Autodesk Inventor part; units mm, degrees
ref_plane "YZ Plane" through (0, 0, 0) normal (1, 0, 0) x (0, 1, 0)
ref_plane "XZ Plane" through (0, 0, 0) normal (0, 1, 0) x (-1, 0, 0)
ref_plane "XY Plane" through (0, 0, 0) normal (0, 0, 1) x (1, 0, 0)
sketch "Sketch1" plane through (0, 0, 0) normal (0, 0, 1) x (1, 0, 0)
  line L0 (0, 0) -> (25.4, 0)
  line L1 (25.4, 0) -> (25.4, 25.4)
  line L2 (25.4, 25.4) -> (0, 25.4)
  line L3 (0, 25.4) -> (0, 0)
  circle A0 centre (12.7, 12.7) radius 3.175
  dimension "d0" = 25.4
  dimension "d1" = 25.4
  dimension "d2" = 6.35
  dimension "d7" = 12.7
  dimension "d8" = 12.7
extrude "Extrusion1" add sketch "Sketch1" along normal blind 609.6
sketch "Sketch2" plane through (0, 0, 609.6) normal (0, 0, 1) x (1, 0, 0)
  line L0 (25.4, 25.4) -> (0, 25.4)
  line L1 (0, 25.4) -> (0, 0)
  circle A0 centre (12.7, 12.7) radius 3.175
  line L2 (0, 0) -> (25.4, 0)
  line L3 (25.4, 0) -> (25.4, 25.4)
  line L4 (25.4, 25.4) -> (0, 25.4)
  line L5 (0, 25.4) -> (0, 0)
  line L6 (12.7, 19.05) -> (9.525, 19.05)
  line L7 (9.525, 19.05) -> (15.875, 19.05)
  line L8 (15.875, 19.05) -> (19.05, 25.4)
  line L9 (9.525, 19.05) -> (6.35, 25.4)
  dimension "d13" = 6.35
  dimension "d14" = 6.35
  dimension "d15" = 3.175
  dimension "d16" = 6.35
fillet "Fillet1" radius 1.5875 4 edges at (25.4, 25.4, 304.8) (0, 25.4, 304.8) (25.4, 0, 304.8) (0, 0, 304.8)
extrude "Extrusion2" cut sketch "Sketch2" against normal blind 609.6 contours L8 L7 L6 L9 L0
pattern_circular "Circular Pattern1" count 4 over 360 about axis through (12.7, 12.7, 0) along (0, 0, 1) of "Extrusion2"
sketch "Sketch3" plane through (0, 0, 609.6) normal (0, 0, 1) x (1, 0, 0)
  line L0 (19.05, 15.875) -> (25.4, 19.05)
  line L1 (25.4, 19.05) -> (25.4, 23.8125)
  arc A0 (25.4, 23.8125) -> (23.8125, 25.4) centre (23.8125, 23.8125) ccw
  line L2 (23.8125, 25.4) -> (19.05, 25.4)
  line L3 (19.05, 25.4) -> (15.875, 19.05)
  line L4 (15.875, 19.05) -> (9.525, 19.05)
  line L5 (9.525, 19.05) -> (6.35, 25.4)
  line L6 (6.35, 25.4) -> (1.5875, 25.4)
  arc A1 (1.5875, 25.4) -> (0, 23.8125) centre (1.5875, 23.8125) ccw
  line L7 (0, 23.8125) -> (0, 19.05)
  line L8 (0, 19.05) -> (6.35, 15.875)
  line L9 (6.35, 15.875) -> (6.35, 9.525)
  line L10 (6.35, 9.525) -> (0, 6.35)
  line L11 (0, 6.35) -> (0, 1.5875)
  arc A2 (0, 1.5875) -> (1.5875, 0) centre (1.5875, 1.5875) ccw
  line L12 (1.5875, 0) -> (6.35, 0)
  line L13 (6.35, 0) -> (9.525, 6.35)
  line L14 (9.525, 6.35) -> (15.875, 6.35)
  line L15 (15.875, 6.35) -> (19.05, 0)
  line L16 (19.05, 0) -> (23.8125, 0)
  arc A3 (23.8125, 0) -> (25.4, 1.5875) centre (23.8125, 1.5875) ccw
  line L17 (25.4, 1.5875) -> (25.4, 6.35)
  line L18 (25.4, 6.35) -> (19.05, 9.525)
  line L19 (19.05, 9.525) -> (19.05, 15.875)
  circle A4 centre (12.7, 12.7) radius 3.175
  point P0 (0, 0)
extrude "Extrusion3" cut sketch "Sketch3" against normal blind 517.525
properties part number "Mock 8020 3.625in"
Design review of the part built by this model. Coordinates are the model's own, in mm. A direction names the side the tool comes from. Round coordinates to 2 decimals unless told otherwise and drop trailing zeros. Loops run counter-clockwise (first coordinate to the right, second up) from the corner with the lowest first, then second, coordinate; pieces in that order, holes last. Notation, with made-up numbers: (-35, -5.5) - (-16, -5.5) arc R18 cw to (-16, 9.5) - close; hole circle Ø4 at (47, -10.5). An arc over 180 degrees is marked (long way). One line per item, written item: value. Start each with the question number.
1) Insertion check: pin 1 Ø5 at (x, z) = (14, 30.5) entering from -Y; pin 2 Ø1.9 at (y, z) = (11.5, 53.5) entering from +X; pin 3 Ø1 at (x, z) = (7, 21.5) entering from -Y; pin 4 Ø3 at (x, z) = (3.5, 51.5) entering from -Y. Each pin has a flat end and moves straight along its axis. Give the tip position at first contact, or say it passes through.
2) Consider section A-A on y = 21. Give the boundary of the cut face in (x, z) (3 decimals), then the cut area to 3 significant figures.
3) To check wall thickness, follow L1, parallel to Y at x = 12.7, z = 58.5 (3 decimals); L2, parallel to X at y = 6, z = 86.5; L3, parallel to Y at x = 15.5, z = 41.5. State the ranges of each line that lie inside material, in increasing order. Write a range as from..to.
4) Consider section C-C on x = 12.7. Give the boundary of the cut face in (y, z) (3 decimals).
5) For faces 1 (the flat face through (3.22, 17.44, 46.68)), 2 (the flat face through (0, 4, 45)), 3 (the flat face through (7.96, 22.18, 46.68)), 4 (the flat face through (19.05, 13, 47)), list the 3-axis set-ups (+Z, -Z, +X, -X, +Y, -Y) from which the entire face can be reached by the end or side of a thin tool; tool diameter is ignored.
6) Consider section D-D on y = 7.5. Give the boundary of the cut face in (x, z) (3 decimals), then the cut area to 3 significant figures.
7) Draft analysis for pull direction X (two halves, no side actions). For faces 5 (the flat face through (0, 21, 45)), 6 (the flat face through (4, 25.4, 45)), 7 (the flat face through (17.44, 3.22, 46.68)), state which applies: +X half, -X half, draft (parallel to the pull), parting line (faces both ways), or undercut.
Reported:
1. pin 1: stops at y = 5.1
1. pin 2: stops at x = 19.05
1. pin 3: stops at y = 0.3
1. pin 4: stops at y = 0
2. outline: (0, 0) - (8.55, 0) - (8.55, 92.075) - (0, 92.075) - close; (16.85, 0) - (25.4, 0) - (25.4, 92.075) - (16.85, 92.075) - close
2. area: 1,570 mm^2
3. L1: y = 6.35..9.525, 15.875..19.05
3. L2: x = 0..9.35, 16.05..25.4
3. L3: y = 6.35..11.2, 14.2..19.05
4. outline: (6.35, 0) - (9.525, 0) - (9.525, 92.075) - (6.35, 92.075) - close; (15.875, 0) - (19.05, 0) - (19.05, 92.075) - (15.875, 92.075) - close
5. face 1: +Z, -Z, -X
5. face 2: +Z, -Z, -X, +Y, -Y
5. face 3: +Z, -Z, +Y
5. face 4: +Z, -Z, +X
6. outline: (2.3, 0) - (23.1, 0) - (23.1, 92.075) - (2.3, 92.075) - close
6. area: 1,920 mm^2
7. face 5: -X half
7. face 6: draft
7. face 7: undercut
